from build123d import *

# Parameters (mm, degrees)
F2_DEPTH = 76.2
F1_W     = 21.9710022211
F1_H     = 51.1809997261
F3_DEPTH = 127
F1_W_2   = 24.3839994073
F4_DEPTH = 127
F5_DEPTH = 25.4
F6_DEPTH = 25.4


with BuildPart() as f2:
    # F0 (on Front) → F2 (new body)
    with BuildSketch(Plane.XZ):
        Polygon((-152.4, 0), (0, 0), (0, 25.4), (-127, 25.4), (-127, 50.8), (-152.4, 50.8), align=None)
        Polygon((-127, 25.4), (0, 25.4), (-127, 50.8), align=None)
    extrude(amount=-F2_DEPTH)

    # F1 (on Right) → F3 (join)
    with BuildSketch(Plane.YZ):
        with Locations((10.9855011106, 25.590499863)):
            Rectangle(F1_W, F1_H)
    extrude(amount=-F3_DEPTH)

    # F1 (on Right) → F4 (join)
    with BuildSketch(Plane.YZ):
        with Locations((63.6270008981, 25.590499863)):
            Rectangle(F1_W_2, F1_H)
    extrude(amount=-F4_DEPTH)

    # F5 (cut): faces of the model
    f5_faces = [f2.faces().sort_by_distance(p)[0] for p in [
        (-63.5, 10.9855011106, 51.1809997261),
        (-63.5, 63.6270008981, 51.1809997261),
    ]]
    extrude(f5_faces, amount=-F5_DEPTH, mode=Mode.SUBTRACT)

    # F6 (cut): a face of the model
    f6_faces = [f2.faces().sort_by_distance(p)[0] for p in [
        (-85.3016662101, 75.8190006018, 34.120666484),
    ]]
    extrude(f6_faces, amount=-F6_DEPTH, mode=Mode.SUBTRACT)


solid = f2.part
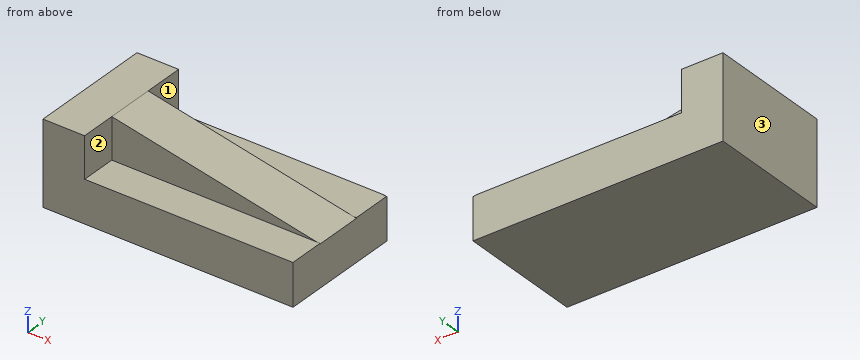
Design review of the part built by this model. Coordinates are the model's own, in mm. Face numbers are marked on the shaded views. A direction names the side the tool comes from. Round coordinates to 2 decimals unless told otherwise and drop trailing zeros. Loops run counter-clockwise (first coordinate to the right, second up) from the corner with the lowest first, then second, coordinate; pieces in that order, holes last. Notation, with made-up numbers: (40.25, -34.75) -> (81.25, -34.75) arc R18 ccw to (81.25, -3.75) -> close; hole circle Ø10 at (23, 14.25). An arc over 180 degrees is marked (long way). Use one line per item in the form item = value. Start each with the question number.
Q1. We need section B-B on x = -44. Give the boundary of the cut face in (y, z) (3 decimals).
Q2. We need section D-D on y = 12.5. Give the boundary of the cut face in (x, z).
Q3. Machinability: for the marked faces 1, 2 and 3, which of the approach directions +Z, -Z, +X, -X, +Y, -Y give a long, thin tool a straight path to every point of the face, cutting with its end or side? Answer none if there is none.
Q4. For pin 1 Ø3 at (x, z) = (-45.5, 34) entering from -Y; pin 2 Ø7.5 at (x, z) = (-80, 44) entering from +Y (3 decimals); pin 3 Ø6.5 at (y, z) = (6.5, 41) entering from +X; pin 4 Ø4 at (y, z) = (35.5, 21.5) entering from +X, all flat-tipped, find the tip position at first contact; note any pin that passes through.
Q5. Wall thickness on line 1 along Z through (x, y) = (-67, 51.5); line 2 along X through (y, z) = (66.5, 28); line 3 along Y through (x, z) = (-122.5, 37) (3 decimals): over which ranges is each line inside the solid? List them lowest first. Write a range as [from, to].
Q6. We need section C-C on y = 26.5. Give the boundary of the cut face in (x, z).
Q7. We need section A-A on z = 47. Give the boundary of the cut face in (x, y) (3 decimals).
Calculated:
q1.outline = (0, 0) -> (76.2, 0) -> (76.2, 25.781) -> (51.435, 25.781) -> (51.435, 34.2) -> (21.971, 34.2) -> (21.971, 25.781) -> (0, 25.781) -> close
q2.outline = (-152.4, 0) -> (0, 0) -> (0, 25.78) -> (-127, 25.78) -> (-127, 50.8) -> (-152.4, 50.8) -> close
q3.face_1 = +Z, +X, +Y
q3.face_2 = +Z, +X, -Y
q3.face_3 = +Z, -Z, -X, +Y, -Y
q4.pin_1 = 21.97
q4.pin_2 = 51.435
q4.pin_3 = -127
q4.pin_4 = 0
q5.line_1 = [0, 25.78]
q5.line_2 = [-152.4, -127]
q5.line_3 = [21.971, 51.435]
q6.outline = (-152.4, 0) -> (0, 0) -> (0, 25.4) -> (-127, 50.8) -> (-152.4, 50.8) -> close
q7.outline = (-152.4, 0) -> (-127, 0) -> (-127, 21.971) -> (-108, 21.971) -> (-108, 51.435) -> (-127, 51.435) -> (-127, 76.2) -> (-152.4, 76.2) -> close
